from build123d import *

# Parameters (mm, degrees)
SKETCH1_R           = 3
SKETCH1_R_2         = 2
SKETCH1_R_3         = 1.25
BOSS_EXTRUDE1_DEPTH = 2
BOSS_EXTRUDE3_DEPTH = 2


with BuildPart() as part:
    # Sketch1 → Boss-Extrude1 (new body)
    with BuildSketch(Plane(origin=(0, 0, 0), x_dir=(0, 0, -1), z_dir=(1, 0, 0))):
        with BuildLine():
            Line((0, 0), (110, 0))
            ThreePointArc((110, 0), (115, 5), (110, 10))
            Line((110, 10), (0, 10))
            ThreePointArc((0, 10), (-5, 5), (0, 0))
        make_face()
        with Locations((0, 5)):
            Circle(SKETCH1_R, mode=Mode.SUBTRACT)
        with Locations((110, 5)):
            Circle(SKETCH1_R_2, mode=Mode.SUBTRACT)
        with Locations((90, 5)):
            Circle(SKETCH1_R_3, mode=Mode.SUBTRACT)
    extrude(amount=BOSS_EXTRUDE1_DEPTH)

    # Sketch2 → Boss-Extrude3 (add)
    with BuildSketch(Plane(origin=(2, 0, 0), x_dir=(0, 0, -1), z_dir=(1, 0, 0))):
        with BuildLine():
            Line((0, 0), (110, 0))
            ThreePointArc((110, 0), (115, 5), (110, 10))
            Line((110, 10), (0, 10))
            ThreePointArc((0, 10), (-5, 5), (0, 0))
        make_face()
        with BuildLine():
            Line((0, 9.25), (110, 9.25))
            ThreePointArc((110, 9.25), (114.25, 5), (110, 0.75))
            Line((110, 0.75), (0, 0.75))
            ThreePointArc((0, 0.75), (-4.25, 5), (0, 9.25))
        make_face(mode=Mode.SUBTRACT)
    extrude(amount=BOSS_EXTRUDE3_DEPTH)


solid = part.part
Model file for the job. Use its own axes, mm. A direction names the side the tool comes from. Give positions to 0.01 mm unless a question says otherwise; leave off trailing zeros. Order: outer loops, then holes, each group sorted by start corner. A loop starts at its lowest first (then second) coordinate and runs counter-clockwise, first axis right, second up. Notation, with made-up numbers: M 7,42.5 L 32,42.5 A29 cw 32,79.5 Z; hole C 11,27 d5. An arc over 180 degrees is marked long. Put each result on its own line as item: value. Start each with the question number.
(1) Band-saw the part on C-C on y = 5. Give the cut face in (x, z), then the cut area to 3 significant figures.
(2) Pin check, flat tips, straight feed: pin 1 Ø1.5 at (x, y) = (2.5, 4) entering from -Z; pin 2 Ø1.5 at (y, z) = (7, -79) entering from +X. Stop position of each tip, or through.
(3) Band-saw the part on A-A on x = 0.95. Give the cut face in (y, z).
(4) Band-saw the part on B-B on z = -90. Give the cut face in (x, y), then the cut area to 3 significant figures.
(5) Pull direction Y, two halves, no side cores. Call faces 1 (the face through (2, 5, -115)), 2 (the face through (2.99, 4.91, 4.25)), 3 (the face through (0, 5, -54)), 4 (the face through (0.986, 4.521, -91.155)): released by +Y, released by -Y, zero draft, split by the parting line, or undercut.
(6) Drill centre lines: L1, parallel to Y at x = 1.05, z = -90; L2, parallel to Z at x = 1.4, y = 6.5; L3, parallel to Y at x = 2.85, z = -10.5. Where is each one in solid material? Low to high. Write a range as [from, to].
(7) Tool access for faces 5 (the face through (2.99, 5.09, -114.25)), 6 (the face through (4, 9.5, -54.7)): list every direction of +Z, -Z, +X, -X, +Y, -Y with a clear straight run to the whole face (end or side of a thin tool).
(8) Band-saw the part on D-D on z = -13. Give the cut face in (x, y).
Results below:
1. outline: M 0,-115 L 4,-115 L 4,-114.25 L 2,-114.25 L 2,-112 L 0,-112 Z; M 0,-108 L 2,-108 L 2,-91.25 L 0,-91.25 Z; M 0,-88.75 L 2,-88.75 L 2,-3 L 0,-3 Z; M 0,3 L 2,3 L 2,4.25 L 4,4.25 L 4,5 L 0,5 Z
1. area: 218 mm2
2. pin 1: stops at z = -114.99
2. pin 2: stops at x = 2
3. outline: M 0,-110 A5 ccw 10,-110 L 10,0 A5 ccw 0,0 Z; hole C 5,0 d6; hole C 5,-110 d4; hole C 5,-90 d2.5
4. outline: M 0,0 L 4,0 L 4,0.75 L 2,0.75 L 2,3.75 L 0,3.75 Z; M 0,6.25 L 2,6.25 L 2,9.25 L 4,9.25 L 4,10 L 0,10 Z
4. area: 18.0 mm2
5. face 1: split by the parting line
5. face 2: undercut
5. face 3: zero draft
5. face 4: undercut
6. L1: y = [0, 3.75], [6.25, 10]
6. L2: z = [-114.77, -111.32], [-108.68, -2.6], [2.6, 4.77]
6. L3: y = [0, 0.75], [9.25, 10]
7. face 5: +X
7. face 6: +Z, -Z, +X, +Y, -Y
8. outline: M 0,0 L 4,0 L 4,0.75 L 2,0.75 L 2,9.25 L 4,9.25 L 4,10 L 0,10 Z
